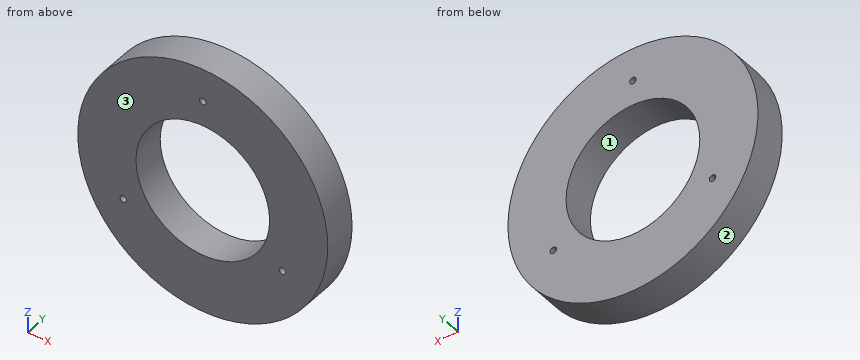
```python
from build123d import *

# Parameters (mm, degrees)
F0_R     = 4.760132
F2_DEPTH = 1.27
F1_R     = 2.546317
F3_DEPTH = 12.7
F4_R     = 0.123894
F5_DEPTH = 25.4


with BuildPart() as f2:
    # F0 (on Front) → F2 (new body)
    with BuildSketch(Plane.XZ):
        Circle(F0_R)
    extrude(amount=F2_DEPTH)

    # F1 (on face) → F3 (cut)
    with BuildSketch(Plane.XZ):
        Circle(F1_R)
    extrude(amount=F3_DEPTH, mode=Mode.SUBTRACT)

    # F4 (on face) → F5 (cut)
    with BuildSketch(Plane.XZ.offset(1.27)):
        with Locations((0, 3.499863)):
            Circle(F4_R)
        with Locations((-3.03097, -1.749931)):
            Circle(F4_R)
        with Locations((3.03097, -1.749931)):
            Circle(F4_R)
    extrude(amount=-F5_DEPTH, mode=Mode.SUBTRACT)


solid = f2.part
```
The listing builds one solid part. Answer for the finished solid, in the listing's coordinates (mm). Face numbers are marked on the shaded views. Coordinates: 2 decimals unless noted, no trailing zeros. Order: outer loops, then holes, each group sorted by start corner. A loop starts at its lowest first (then second) coordinate and runs counter-clockwise, first axis right, second up. Notation, with made-up numbers: M -24.5,-9.5 L -19.5,-9.5 A12 ccw -19.5,9.5 Z; hole C 3,1 d2. An arc over 180 degrees is marked long. Answer as a JSON object with one key per item and string values. Group by question number.
1. Section D-D on y = -0.2 is taken. Write down the section's boundary in (x, z), then the cut area to 3 significant figures.
2. Section B-B on z = 0 is taken. Write down the section's boundary in (x, y).
3. Straight lines are drawn through the part: line 1 (Z direction, x = 0, y = -0.6); line 2 (X direction, y = -0.6, z = -1.75); line 3 (Z direction, x = 0.25, y = -0.65). For each, find the intervals that lie inside material, in ascending order.
4. Section C-C on x = 1.5 is taken. Write down the section's boundary in (y, z), then the cut area to 3 significant figures.
5. Section A-A on x = 0 is taken. Write down the section's boundary in (y, z), then the cut area to 3 significant figures.
6. Determine the mould class of the marked faces 1, 2 and 3 for opening direction Z: released by +Z, released by -Z, zero draft, split by the parting line, or undercut.
Values follow:
{
 "1": {"outline": "C 0,0 d9.52; hole C -3.03,-1.75 d0.25; hole C 0,0 d5.09; hole C 0,3.5 d0.25; hole C 3.03,-1.75 d0.25", "area": "50.7 mm2"},
 "2": {"outline": "M -4.76,-1.27 L -2.55,-1.27 L -2.55,0 L -4.76,0 Z; M 2.55,-1.27 L 4.76,-1.27 L 4.76,0 L 2.55,0 Z"},
 "3": {"line 1": "-4.76 to -2.55, 2.55 to 3.38, 3.62 to 4.76", "line 2": "-4.43 to -3.15, -2.91 to -1.85, 1.85 to 2.91, 3.15 to 4.43", "line 3": "-4.75 to -2.53, 2.53 to 4.75"},
 "4": {"outline": "M -1.27,-4.52 L 0,-4.52 L 0,-2.06 L -1.27,-2.06 Z; M -1.27,2.06 L 0,2.06 L 0,4.52 L -1.27,4.52 Z", "area": "6.25 mm2"},
 "5": {"outline": "M -1.27,-4.76 L 0,-4.76 L 0,-2.55 L -1.27,-2.55 Z; M -1.27,2.55 L 0,2.55 L 0,3.38 L -1.27,3.38 Z; M -1.27,3.62 L 0,3.62 L 0,4.76 L -1.27,4.76 Z", "area": "5.31 mm2"},
 "6": {"face 1": "undercut", "face 2": "split by the parting line", "face 3": "zero draft"}
}
